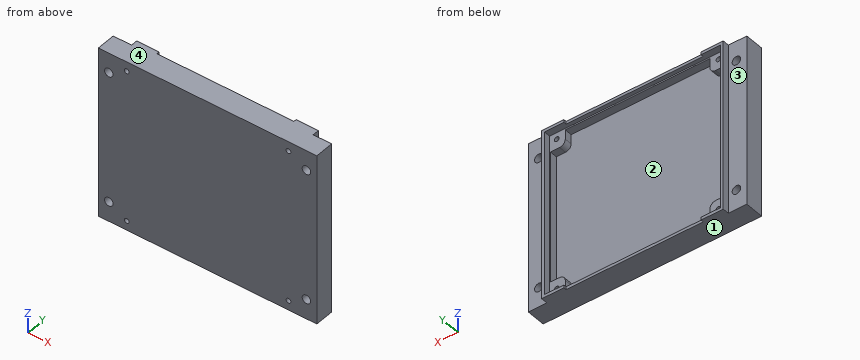
```python
from build123d import *

# Parameters (mm, degrees)
SKETCH1_W           = 115.5
SKETCH1_H           = 90.5
BOSS_EXTRUDE1_DEPTH = 10
SKETCH2_W           = 96
SKETCH2_H           = 90.5
SKETCH2_W_2         = 93
SKETCH2_H_2         = 87.5
BOSS_EXTRUDE2_DEPTH = 3.5
SKETCH3_R           = 1.25
CUT_EXTRUDE1_DEPTH  = 20
CUT_EXTRUDE2_DEPTH  = 4
FILLET1_R           = 3
SKETCH5_R           = 2.25
CUT_EXTRUDE3_DEPTH  = 15
SKETCH6_W           = 72.5
SKETCH6_H           = 10.501850212
CUT_EXTRUDE4_DEPTH  = 98


with BuildPart() as part:
    # Sketch1 → Boss-Extrude1 (new body)
    with BuildSketch(Plane(origin=(0, 0, 0), x_dir=(1, 0, 0), z_dir=(0, 1, 0))):
        Rectangle(SKETCH1_W, SKETCH1_H)
    extrude(amount=BOSS_EXTRUDE1_DEPTH)

    # Sketch2 → Boss-Extrude2 (add)
    with BuildSketch(Plane(origin=(0, 10, 0), x_dir=(1, 0, 0), z_dir=(0, 1, 0))):
        Rectangle(SKETCH2_W, SKETCH2_H)
        Rectangle(SKETCH2_W_2, SKETCH2_H_2, mode=Mode.SUBTRACT)
    extrude(amount=BOSS_EXTRUDE2_DEPTH)

    # Sketch3 → Cut-Extrude1 (cut)
    with BuildSketch(Plane(origin=(0, 10, 0), x_dir=(1, 0, 0), z_dir=(0, 1, 0))):
        with Locations(Location((-42.75, 40.25, 0), (0, 0, 270))):
            Circle(SKETCH3_R)
        with Locations(Location((42.75, 40.25, 0), (0, 0, 270))):
            Circle(SKETCH3_R)
        with Locations(Location((42.75, -40.25, 0), (0, 0, 270))):
            Circle(SKETCH3_R)
        with Locations(Location((-42.75, -40.25, 0), (0, 0, 270))):
            Circle(SKETCH3_R)
    extrude(amount=-CUT_EXTRUDE1_DEPTH, mode=Mode.SUBTRACT)

    # Sketch4 → Cut-Extrude2 (cut)
    with BuildSketch(Plane(origin=(0, 10, 0), x_dir=(1, 0, 0), z_dir=(0, 1, 0))):
        Polygon((-38.25, 42.95), (38.25, 42.95), (38.25, 35), (46.1, 35), (46.1, -35), (38.25, -35), (38.25, -42.95), (-38.25, -42.95), (-38.25, -35), (-46.1, -35), (-46.1, 35), (-38.25, 35), align=None)
    extrude(amount=-CUT_EXTRUDE2_DEPTH, mode=Mode.SUBTRACT)

    # Fillet1
    fillet1_edges = [part.edges().sort_by_distance(p)[0] for p in [
        (-38.25, 8, -35),
        (38.25, 8, -35),
        (38.25, 8, 35),
        (-38.25, 8, 35),
    ]]
    fillet(fillet1_edges, radius=FILLET1_R)

    # Sketch5 → Cut-Extrude3 (cut)
    with BuildSketch(Plane(origin=(0, 10, 0), x_dir=(1, 0, 0), z_dir=(0, 1, 0))):
        with Locations(Location((-52.25, 34.75, 0), (0, 0, 270))):
            Circle(SKETCH5_R)
        with Locations(Location((52.25, 34.75, 0), (0, 0, 270))):
            Circle(SKETCH5_R)
        with Locations(Location((52.25, -34.75, 0), (0, 0, 270))):
            Circle(SKETCH5_R)
        with Locations(Location((-52.25, -34.75, 0), (0, 0, 270))):
            Circle(SKETCH5_R)
    extrude(amount=-CUT_EXTRUDE3_DEPTH, mode=Mode.SUBTRACT)

    # Sketch6 → Cut-Extrude4 (cut)
    with BuildSketch(Plane.XY.offset(45.25)):
        with Locations((0, 17.250925106)):
            Rectangle(SKETCH6_W, SKETCH6_H)
    extrude(amount=-CUT_EXTRUDE4_DEPTH, mode=Mode.SUBTRACT)


solid = part.part
```
Here's how the part is built. I have some questions about the finished solid (model axes, mm). Face numbers are marked on the shaded views. A direction names the side the tool comes from. Coordinates: 2 decimals unless noted, no trailing zeros. Loops run counter-clockwise (first coordinate to the right, second up) from the corner with the lowest first, then second, coordinate; pieces in that order, holes last. Notation, with made-up numbers: (72, 88.5) -> (88, 88.5) arc R30 cw to (88, 119.5) -> close; hole circle Ø4 at (-6, -35.75). An arc over 180 degrees is marked (long way). Return JSON: item names as keys, results as strings.
1) For the marked faces 3 and 4, which set-ups out of +Z, -Z, +X, -X, +Y, -Y let a thin tool reach every point of the face, with its end or its side?
Results below:
{"face 3": "+Z, -Z, -X, +Y", "face 4": "+Z, +X, -X, +Y, -Y"}
2) If we section it at C-C, the plane z = -40.25: Write out the boundary of the cut face in (x, y).
Results below:
{"outline": "(-57.75, 0) -> (-44, 0) -> (-44, 10) -> (-46.5, 10) -> (-46.5, 13.5) -> (-48, 13.5) -> (-48, 10) -> (-57.75, 10) -> close; (-41.5, 0) -> (41.5, 0) -> (41.5, 10) -> (38.25, 10) -> (38.25, 6) -> (-38.25, 6) -> (-38.25, 10) -> (-41.5, 10) -> close; (44, 0) -> (57.75, 0) -> (57.75, 10) -> (48, 10) -> (48, 13.5) -> (46.5, 13.5) -> (46.5, 10) -> (44, 10) -> close"}
3) If we section it at D-D, the plane x = -22.5: Write out the boundary of the cut face in (y, z).
Results below:
{"outline": "(0, -45.25) -> (12, -45.25) -> (12, -43.75) -> (10, -43.75) -> (10, -42.95) -> (6, -42.95) -> (6, 42.95) -> (10, 42.95) -> (10, 43.75) -> (12, 43.75) -> (12, 45.25) -> (0, 45.25) -> close"}
4) If we section it at A-A, the plane x = 52.25: Write out the boundary of the cut face in (y, z), then the cut area to 3 significant figures.
Results below:
{"outline": "(0, -45.25) -> (10, -45.25) -> (10, -37) -> (0, -37) -> close; (0, -32.5) -> (10, -32.5) -> (10, 32.5) -> (0, 32.5) -> close; (0, 37) -> (10, 37) -> (10, 45.25) -> (0, 45.25) -> close", "area": "815 mm²"}
5) If we section it at B-B, the plane y = 8: Count the separate pieces of the cut face and the enclosed holes in it, then the cut area to 3 significant figures.
Results below:
{"separate pieces": "1", "enclosed holes": "9", "area": "2,690 mm²"}
6) Thinking about a two-plate mould opening in X: for the marked faces 1 and 2, which applies, +X half, -X half, draft (parallel to the pull), parting line (faces both ways), or undercut?
Results below:
{"face 1": "draft", "face 2": "undercut"}
7) Will these pins go through, and if not, where does the flat tip stop? pin 1 (10 mm diameter, centred on x = 2, z = 14, fed in from +Y); pin 2 (1.2 mm diameter, centred on y = 12.5, z = 44.5, fed in from +X); pin 3 (4 mm diameter, centred on x = -52.25, z = 34.75, fed in from -Y); pin 4 (0.8 mm diameter, centred on x = -12, z = 44, fed in from +Y).
Results below:
{"pin 1": "y = 6", "pin 2": "x = 48", "pin 3": "through", "pin 4": "y = 12"}
8) I need wall thicknesses on line 1 (X direction, y = 9.25, z = 40); line 2 (Z direction, x = 52, y = 3); line 3 (X direction, y = 4, z = -34.75). Which ranges of each line are inside material? Lowest first, please. Write a range as from..to.
Results below:
{"line 1": "-57.75..-43.97, -41.53..-38.25, 38.25..41.53, 43.97..57.75", "line 2": "-45.25..-36.99, -32.51..32.51, 36.99..45.25", "line 3": "-57.75..-54.5, -50..50, 54.5..57.75"}
